CAD build for the part. Positions are in the model's coordinates, mm. A direction names the side the tool comes from. Round coordinates to 2 decimals unless told otherwise and drop trailing zeros. Order: outer loops, then holes, each group sorted by start corner. A loop starts at its lowest first (then second) coordinate and runs counter-clockwise, first axis right, second up. Notation, with made-up numbers: M 9.5,66.5 L 60.5,66.5 A26 cw 60.5,97.5 Z; hole C -9,24.25 d5. An arc over 180 degrees is marked long. Answer as a JSON object with one key per item and string values.
```python
from build123d import *

# Parameters (mm, degrees)
F0_W     = 15.875
F0_H     = 15.875
F1_DEPTH = 4.7625
F2_R     = 2.4511
F3_DEPTH = 1.778
F4_W     = 13.589
F4_H     = 13.589
F4_R     = 3.2385
F5_DEPTH = 8.382
F6_R     = 2.4765
F7_DEPTH = 8.382


with BuildPart() as f1:
    # F0 (on Top) → F1 (new body, symmetric)
    with BuildSketch(Plane.XY):
        Rectangle(F0_W, F0_H)
    extrude(amount=F1_DEPTH, both=True)

    # F2 (on face) → F3 (join)
    with BuildSketch(Plane.XY.offset(4.7625)):
        with Locations((-4.0132, -4.0132)):
            Circle(F2_R)
        with Locations((4.0132, -4.0132)):
            Circle(F2_R)
        with Locations((4.0132, 4.0132)):
            Circle(F2_R)
        with Locations((-4.0132, 4.0132)):
            Circle(F2_R)
    extrude(amount=F3_DEPTH)

    # F4 (on face) → F5 (cut)
    with BuildSketch(Plane(origin=(0, 0, -4.7625), x_dir=(1, 0, 0), z_dir=(0, 0, -1))):
        Rectangle(F4_W, F4_H)
        Circle(F4_R, mode=Mode.SUBTRACT)
    extrude(amount=-F5_DEPTH, mode=Mode.SUBTRACT)

    # F6 (on face) → F7 (cut)
    with BuildSketch(Plane(origin=(0, 0, -4.7625), x_dir=(1, 0, 0), z_dir=(0, 0, -1))):
        Circle(F6_R)
    extrude(amount=-F7_DEPTH, mode=Mode.SUBTRACT)


solid = f1.part
```
Item 1: Saw through at D-D on z = 5.5. List the corners of the cut face in (x, y).
Worked answers:
{"outline": "C -4.01,-4.01 d4.9; C -4.01,4.01 d4.9; C 4.01,-4.01 d4.9; C 4.01,4.01 d4.9"}
Item 2: Two-plate mould, pull along Y, no slides. Class faces 4 (the flat face through (0, -7.938, 0)), 5 (the flat face through (0, 7.938, 0)), 6 (the flat face through (0, 0, 4.762)), 7 (the flat face through (4, -4, 6.54)): released by +Y, released by -Y, zero draft, split by the parting line, or undercut.
Worked answers:
{"face 4": "released by -Y", "face 5": "released by +Y", "face 6": "undercut", "face 7": "zero draft"}
Item 3: Saw through at B-B on x = 0. List the corners of the cut face in (y, z), and give its area (3 significant figures).
Worked answers:
{"outline": "M -7.94,-4.76 L -6.79,-4.76 L -6.79,3.62 L -3.24,3.62 L -3.24,-4.76 L -2.48,-4.76 L -2.48,3.62 L 2.48,3.62 L 2.48,-4.76 L 3.24,-4.76 L 3.24,3.62 L 6.79,3.62 L 6.79,-4.76 L 7.94,-4.76 L 7.94,4.76 L -7.94,4.76 Z", "area": "50.1 mm2"}
Item 4: Saw through at C-C on y = -1.25. List the corners of the cut face in (x, z), and give its area (4 significant figures).
Worked answers:
{"outline": "M -7.94,-4.76 L -6.79,-4.76 L -6.79,3.62 L -2.99,3.62 L -2.99,-4.76 L -2.14,-4.76 L -2.14,3.62 L 2.14,3.62 L 2.14,-4.76 L 2.99,-4.76 L 2.99,3.62 L 6.79,3.62 L 6.79,-4.76 L 7.94,-4.76 L 7.94,4.76 L -7.94,4.76 Z", "area": "51.55 mm2"}
Item 5: Saw through at A-A on z = -0.25. List the corners of the cut face in (x, y), and give its area (3 significant figures).
Worked answers:
{"outline": "M -7.94,-7.94 L 7.94,-7.94 L 7.94,7.94 L -7.94,7.94 Z; C 0,0 d6.48; hole M -6.79,-6.79 L 6.79,-6.79 L 6.79,6.79 L -6.79,6.79 Z; hole C 0,0 d4.95", "area": "81.0 mm2"}
Item 6: 3-axis set-ups, long thin cutter, end or side, ignore diameter. For faces 1 (the cylindrical face through (3.694, 6.443, 5.639)), 2 (the flat face through (2, -2, -4.762)), 3 (the flat face through (-6.794, 0, -1)): which of +Z, -Z, +X, -X, +Y, -Y reach the whole face in a straight line?
Worked answers:
{"face 1": "+Z", "face 2": "-Z, +X, -X, +Y, -Y", "face 3": "-Z"}
Item 7: Wall check: line 1 along X through (y, z) = (0, 1.25); line 2 along X through (y, z) = (-5, 0.25). Give the ranges that are in metal, low to high. Write a range as [from, to].
Worked answers:
{"line 1": "x = [-7.94, -6.79], [-3.24, -2.48], [2.48, 3.24], [6.79, 7.94]", "line 2": "x = [-7.94, -6.79], [6.79, 7.94]"}
